Autodesk Inventor part; units mm, degrees
ref_plane "YZ Plane" through (0, 0, 0) normal (1, 0, 0) x (0, 1, 0)
ref_plane "XZ Plane" through (0, 0, 0) normal (0, 1, 0) x (-1, 0, 0)
ref_plane "XY Plane" through (0, 0, 0) normal (0, 0, 1) x (1, 0, 0)
sketch "Эскиз1" plane through (0, 0, 0) normal (0, 1, 0) x (-1, 0, 0)
  line L0 (0, 0) -> (-4, 0)
  line L1 (-4, 29) -> (-4, 60)
  line L2 (-4, 60) -> (0, 60)
  line L3 (0, 60) -> (0, 0)
  line L4 (0, 0) -> (-60, 0)
  line L5 (-60, 0) -> (-60, 4)
  line L6 (-60, 4) -> (-29, 4)
  line L7 (0, 4) -> (0, 0)
  line L8 (-4, 29) -> (-29, 4)
  dimension "d0" = 4
  dimension "d1" = 60
  dimension "d2" = 60
  dimension "d3" = 4
  dimension "d4" = 25
  dimension "d5" = 25
extrude "Выдавливание1" add sketch "Эскиз1" along normal blind 20
sketch "Эскиз2" plane through (4, 0, 60) normal (1, 0, 0) x (0, 0, -1)
  line L0 (0, 20) -> (31, 20)
  line L1 (0, 0) -> (0, 20)
  circle A0 centre (26, 10) radius 2
  line L2 (31, 0) -> (31, 20)
  point P0 (60, 0)
  dimension "d11" = 4
  dimension "d12" = 5
extrude "Выдавливание2" cut sketch "Эскиз2" against normal blind 10
chamfer "Фаска1" distance 1 angle 45 1 edges at (4, 10, 36)
sketch "Эскиз3" plane through (29, 0, 4) normal (0, 0, 1) x (1, 0, 0)
  line L0 (31, 0) -> (31, 20)
  line L1 (31, 20) -> (27, 20)
  line L2 (27, 20) -> (27, 0)
  line L3 (27, 0) -> (31, 0)
  line L4 (31, 0) -> (31, 20)
  line L5 (0, 0) -> (31, 0)
  point P0 (-29, 0)
  point P1 (29, 0)
  dimension "d18" = 4
extrude "Выдавливание3" add sketch "Эскиз3" along normal blind 25
properties part number "corner"
Here's how the part is built. I have some questions about the finished solid (model axes, mm). A direction names the side the tool comes from. Round coordinates to 2 decimals unless told otherwise and drop trailing zeros. Order: outer loops, then holes, each group sorted by start corner. A loop starts at its lowest first (then second) coordinate and runs counter-clockwise, first axis right, second up. Notation, with made-up numbers: M 9.5,2 L 21.5,2 A13 ccw 21.5,20 Z; hole C 61,-25 d5. An arc over 180 degrees is marked long. Return JSON: item names as keys, results as strings. Group by question number.
1. If we mould it in two halves opening along Z, with no side actions, what happens to faces 4 (the face through (16, 10, 17)), 5 (the face through (30, 10, 0)), 6 (the face through (1.521, 10.601, 32.092))? For each: pulls with the +Z half, pulls with the -Z half, needs draft (parallel to the pull), parting line crosses it, or undercut.
2. If we section it at D-D on z = 43: List the corners of the cut face in (x, y) for me, then the cut area to 3 significant figures.
3. On a 3-axis mill with a long thin cutter (end or side, diameter ignored), from which of +Z, -Z, +X, -X, +Y, -Y can I reach the whole of each face in a straight line? I mean faces 1 (the face through (60, 10, 14)), 2 (the face through (4, 10, 44)), 3 (the face through (56, 10, 16)). Say none if no direction works.
4. If we section it at C-C on x = 22.5: List the corners of the cut face in (y, z) for me.
5. If we section it at A-A on y = 15.25: List the corners of the cut face in (x, z) for me, then the cut area to 4 significant figures.
6. If we section it at B-B on z = 34: List the corners of the cut face in (x, y) for me, then the cut area to 3 significant figures.
7. Please list where these lines run through material, in increasing order: probe 1 along Y at (x, z) = (2.1, 34); probe 2 along X at (y, z) = (11.25, 21); probe 3 along X at (y, z) = (15.5, 36.5).
8. I'm going to push flat-ended pins straight in: pin 1 Ø4 at (x, y) = (33, 12.5) entering from +Z; pin 2 Ø3 at (x, y) = (57.5, 13) entering from +Z; pin 3 Ø6.5 at (y, z) = (10, 34) entering from +X. Where does each tip first touch, or does it pass through?
Reply:
{
 "1": {"face 4": "pulls with the +Z half", "face 5": "pulls with the -Z half", "face 6": "undercut"},
 "2": {"outline": "M 0,0 L 4,0 L 4,20 L 0,20 Z", "area": "80.0 mm^2"},
 "3": {"face 1": "+Z, -Z, +X, +Y, -Y", "face 2": "+Z, +X, +Y, -Y", "face 3": "+Z, +Y, -Y"},
 "4": {"outline": "M 0,0 L 20,0 L 20,10.5 L 0,10.5 Z"},
 "5": {"outline": "M 0,0 L 60,0 L 60,29 L 56,29 L 56,4 L 29,4 L 4,29 L 4,60 L 0,60 Z", "area": "876.5 mm^2"},
 "6": {"outline": "M 0,0 L 4,0 L 4,7 L 3,8 L 0,8 Z; M 0,12 L 3,12 L 4,13 L 4,20 L 0,20 Z", "area": "63.0 mm^2"},
 "7": {"probe 1": "0 to 8, 12 to 20", "probe 2": "0 to 12, 56 to 60", "probe 3": "0 to 4"},
 "8": {"pin 1": "z = 4", "pin 2": "z = 29", "pin 3": "x = 4"}
}
